Work out the finished part from the listing and answer in its coordinate system (mm). A direction names the side the tool comes from. Round coordinates to 2 decimals unless told otherwise and drop trailing zeros. Order: outer loops, then holes, each group sorted by start corner. A loop starts at its lowest first (then second) coordinate and runs counter-clockwise, first axis right, second up. Notation, with made-up numbers: (28.5, 82) - (52.5, 82) arc R11 ccw to (52.5, 94) - close; hole circle Ø3 at (9.25, -22). An arc over 180 degrees is marked (long way). Answer in a Markdown table with one row per item.
Autodesk Inventor part; units mm, degrees
ref_plane "YZ Plane" through (0, 0, 0) normal (1, 0, 0) x (0, 1, 0)
ref_plane "XZ Plane" through (0, 0, 0) normal (0, 1, 0) x (-1, 0, 0)
ref_plane "XY Plane" through (0, 0, 0) normal (0, 0, 1) x (1, 0, 0)
sketch "Boceto1" plane through (0, 0, 0) normal (0, 0, 1) x (1, 0, 0)
  line L0 (90, 56) -> (90, -56)
  line L1 (90, -56) -> (64, -56)
  arc A0 (64, -56) -> (60, -56) centre (62, -56) ccw
  line L2 (60, -56) -> (60, -60)
  line L3 (60, -60) -> (20, -60)
  line L4 (20, -60) -> (20, -56)
  arc A1 (20, -56) -> (16, -56) centre (18, -56) ccw
  line L5 (15.6321, 0) -> (-15.6321, 0) construction
  line L6 (0, 12.7826) -> (0, -12.7826) construction
  line L7 (90, 56) -> (64, 56)
  arc A2 (60, 56) -> (64, 56) centre (62, 56) ccw
  line L8 (60, 56) -> (60, 60)
  line L9 (60, 60) -> (20, 60)
  line L10 (20, 60) -> (20, 56)
  arc A3 (16, 56) -> (20, 56) centre (18, 56) ccw
  line L11 (-90, 56) -> (-90, -56)
  line L12 (-90, -56) -> (-64, -56)
  arc A4 (-60, -56) -> (-64, -56) centre (-62, -56) ccw
  line L13 (-60, -56) -> (-60, -60)
  line L14 (-60, -60) -> (-20, -60)
  line L15 (-20, -60) -> (-20, -56)
  arc A5 (-16, -56) -> (-20, -56) centre (-18, -56) ccw
  line L16 (-90, 56) -> (-64, 56)
  arc A6 (-64, 56) -> (-60, 56) centre (-62, 56) ccw
  line L17 (-60, 56) -> (-60, 60)
  line L18 (-60, 60) -> (-20, 60)
  line L19 (-20, 60) -> (-20, 56)
  arc A7 (-20, 56) -> (-16, 56) centre (-18, 56) ccw
  line L20 (-16, 56) -> (16, 56)
  line L21 (-16, -56) -> (16, -56)
  circle A8 centre (0, -48) radius 2
  circle A9 centre (0, 48) radius 2
  circle A10 centre (80, 48) radius 2
  circle A11 centre (80, -48) radius 2
  circle A12 centre (-80, 48) radius 2
  circle A13 centre (-80, -48) radius 2
  point P0 (0, 0)
  point P1 (0, 0)
  dimension "d0" = 2
  dimension "d1" = 120
  dimension "d2" = 40
  dimension "d3" = 4
  dimension "d4" = 40
  dimension "d5" = 30
  dimension "d6" = 8
  dimension "d7" = 4
  dimension "d8" = 20
extrude "Extrusión1" add sketch "Boceto1" along normal blind 4
equation "\"d4\" = d2"
properties part number "bandeja central"
1) Find section B-B, the plane z = 2.15. Give the number of separate pieces and of enclosed holes in the cut face, then the cut area to 3 significant figures.
Filled in:
| item | result |
|---|---|
| separate pieces | 1 |
| enclosed holes | 6 |
| area | 20,700 mm^2 |
2) Find the intervals of material crossed by probe 1 along Y at (x, z) = (80, 2.95); probe 2 along Y at (x, z) = (-79.5, 3.85); probe 3 along X at (y, z) = (-49, 3.05), in increasing order. Write a range as from..to.
Filled in:
| item | result |
|---|---|
| probe 1 | y = -56..-50, -46..46, 50..56 |
| probe 2 | y = -56..-49.94, -46.06..46.06, 49.94..56 |
| probe 3 | x = -90..-81.73, -78.27..-1.73, 1.73..78.27, 81.73..90 |
3) The mould has two halves that part along X. Classify faces 4 (the face through (-1, 1, 4)), 5 (the face through (60, 58, 2)), 6 (the face through (-18, 54, 2)), 7 (the face through (20, 58, 2)): released by +X, released by -X, zero draft, split by the parting line, or undercut.
Filled in:
| item | result |
|---|---|
| face 4 | zero draft |
| face 5 | released by +X |
| face 6 | undercut |
| face 7 | undercut |
4) Find section C-C, the plane y = 48. Give the vertices of the cut face in (x, z).
Filled in:
| item | result |
|---|---|
| outline | (-90, 0) - (-82, 0) - (-82, 4) - (-90, 4) - close; (-78, 0) - (-2, 0) - (-2, 4) - (-78, 4) - close; (2, 0) - (78, 0) - (78, 4) - (2, 4) - close; (82, 0) - (90, 0) - (90, 4) - (82, 4) - close |
5) Find section A-A, the plane x = 0. Give the vertices of the cut face in (y, z).
Filled in:
| item | result |
|---|---|
| outline | (-56, 0) - (-50, 0) - (-50, 4) - (-56, 4) - close; (-46, 0) - (46, 0) - (46, 4) - (-46, 4) - close; (50, 0) - (56, 0) - (56, 4) - (50, 4) - close |
6) Which of the six approach directions +Z, -Z, +X, -X, +Y, -Y give full straight-line access (tool end or side, diameter ignored) to faces 1 (the face through (-20, 58, 2)), 2 (the face through (-77, -56, 2)), 3 (the face through (-60, 58, 2))?
Filled in:
| item | result |
|---|---|
| face 1 | +Z, -Z, +Y |
| face 2 | +Z, -Z, -X, -Y |
| face 3 | +Z, -Z, -X, +Y |
7) Each of these flat-tipped pins is pushed along its axis until it touches: pin 1 (2.5 mm diameter, centred on x = -80, y = -48, fed in from -Z); pin 2 (1.2 mm diameter, centred on x = 71.5, z = 2.5, fed in from -Y); pin 3 (2 mm diameter, centred on x = -17.5, z = 2, fed in from +Y); pin 4 (1.2 mm diameter, centred on x = 77.5, z = 1.5, fed in from +Y). Where does it stop, or does it pass through?
Filled in:
| item | result |
|---|---|
| pin 1 | passes through |
| pin 2 | stops at y = -56 |
| pin 3 | stops at y = 54.68 |
| pin 4 | stops at y = 56 |
8) Find section D-D, the plane x = 62. Give the vertices of the cut face in (y, z), then the cut area to 3 significant figures.
Filled in:
| item | result |
|---|---|
| outline | (-54, 0) - (54, 0) - (54, 4) - (-54, 4) - close |
| area | 432 mm^2 |
